Check sheet for the drawn part. Datum: minimum x, y, z corner. Units: mm. A direction names the side the tool comes from. Round coordinates to 2 decimals unless told otherwise and drop trailing zeros. Order: outer loops, then holes, each group sorted by start corner. A loop starts at its lowest first (then second) coordinate and runs counter-clockwise, first axis right, second up. Notation, with made-up numbers: (47.25, -8.5) -> (69.25, -8.5) arc R18 ccw to (69.25, 26.5) -> close; hole circle Ø6 at (20.5, 59). An arc over 180 degrees is marked (long way). Write item = value, one per line. Start each with the question number.
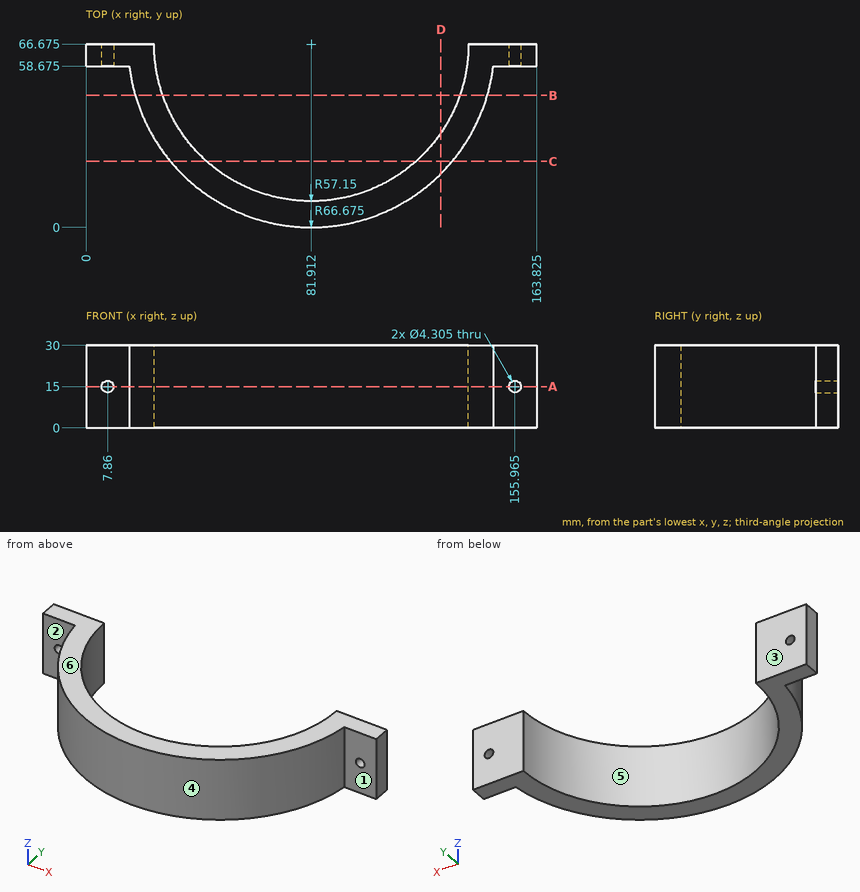
(1) Cross-section at D-D (x = 129). Enter the section's corners in (y, z).
(2) Depth check by flat-ended pin: pin 1 (8 mm diameter, centred on x = 11.5, z = 21, fed in from -Y) (1 decimal); pin 2 (5 mm diameter, centred on x = 34, z = 21.5, fed in from -Y) (1 decimal); pin 3 (8 mm diameter, centred on x = 68.5, z = 20.5, fed in from -Y). Enter the tip coordinate at first touch or a pass-through.
(3) Set-up check for the marked faces 1, 2 and 3: record each of +Z, -Z, +X, -X, +Y, -Y from which the full face is reachable in a straight line by a thin tool's end or side.
(4) Cross-section at A-A (z = 15). Give the number of separate pieces and of enclosed holes in the cut face, and give its area (3 significant figures).
(5) Cross-section at C-C (y = 24). Enter the section's corners in (x, z) (1 decimal).
(6) Cross-section at B-B (y = 48). Enter the section's corners in (x, z) (1 decimal).
(7) Scan lines: line 1 along X through (y, z) = (61.5, 15) (1 decimal); line 2 along X through (y, z) = (62.25, 15) (1 decimal); line 3 along Y through (x, z) = (157, 20.75) (1 decimal). Record each from-to range of solid material in increasing order. Write a range as from..to.
(8) Draft check along X on the marked faces 4, 5 and 6. Enter one of: +X half, -X half, draft (parallel to the pull), parting line (faces both ways), or undercut.
Outcome:
q1.outline = (19.47, 0) -> (34.29, 0) -> (34.29, 30) -> (19.47, 30) -> close
q2.pin_1 = 58.7
q2.pin_2 = 17.9
q2.pin_3 = 0.67
q3.face_1 = +Z, -Z, +X, -Y
q3.face_2 = +Z, -Z, -X, -Y
q3.face_3 = +Z, -Z, +X, -X, +Y
q4.separate_pieces = 3
q4.enclosed_holes = 0
q4.area = 2,030 mm^2
q5.outline = (30.7, 0) -> (43.9, 0) -> (43.9, 30) -> (30.7, 30) -> close; (119.9, 0) -> (133.1, 0) -> (133.1, 30) -> (119.9, 30) -> close
q6.outline = (17.9, 0) -> (27.9, 0) -> (27.9, 30) -> (17.9, 30) -> close; (135.9, 0) -> (145.9, 0) -> (145.9, 30) -> (135.9, 30) -> close
q7.line_1 = 0..5.7, 10..25, 138.8..153.8, 158.1..163.8
q7.line_2 = 0..5.7, 10..24.9, 138.9..153.8, 158.1..163.8
q7.line_3 = 58.7..66.7
q8.face_4 = parting line
q8.face_5 = undercut
q8.face_6 = draft
